from build123d import *

# Parameters (mm, degrees)
SKETCH1_W           = 62
SKETCH1_H           = 46
BOSS_EXTRUDE1_DEPTH = 5
SKETCH2_W           = 2
SKETCH2_H           = 5
SKETCH2_H_2         = 9
SKETCH2_H_3         = 32
SKETCH2_W_2         = 5
SKETCH2_H_4         = 2
BOSS_EXTRUDE2_DEPTH = 8
SKETCH3_W           = 17
SKETCH3_H           = 32
BOSS_EXTRUDE3_DEPTH = 1.5
SKETCH4_W           = 7
SKETCH4_H           = 5
BOSS_EXTRUDE4_DEPTH = 2.5


with BuildPart() as part:
    # Sketch1 → Boss-Extrude1 (new body)
    with BuildSketch(Plane(origin=(0, 0, 0), x_dir=(1, 0, 0), z_dir=(0, 1, 0))):
        with Locations((4.368421053, -7.717105263)):
            Rectangle(SKETCH1_W, SKETCH1_H)
    extrude(amount=BOSS_EXTRUDE1_DEPTH)

    # Sketch2 → Boss-Extrude2 (add)
    with BuildSketch(Plane(origin=(0, 5, 0), x_dir=(1, 0, 0), z_dir=(0, 1, 0))):
        with Locations((-20.631578947, 3.782894737)):
            Rectangle(SKETCH2_W, SKETCH2_H)
        with Locations((-20.631578947, -19.217105263)):
            Rectangle(SKETCH2_W, SKETCH2_H)
        Polygon((7.368421053, -23.717105263), (8.368421053, -22.717105263), (2.368421053, -16.717105263), (1.368421053, -17.717105263), align=None)
        with Locations((30.368421053, 6.782894737)):
            Rectangle(SKETCH2_W, SKETCH2_H_2)
        with Locations((30.368421053, -7.717105263)):
            Rectangle(SKETCH2_W, SKETCH2_H_2)
        with Locations((30.368421053, -22.217105263)):
            Rectangle(SKETCH2_W, SKETCH2_H_2)
        with Locations((10.368421053, -7.717105263)):
            Rectangle(SKETCH2_W, SKETCH2_H_3)
        with Locations((25.368421053, -7.717105263)):
            Rectangle(SKETCH2_W, SKETCH2_H_3)
        with Locations((-6.131578947, -24.717105263)):
            Rectangle(SKETCH2_W_2, SKETCH2_H_4)
    extrude(amount=BOSS_EXTRUDE2_DEPTH)

    # Sketch3 → Boss-Extrude3 (add)
    with BuildSketch(Plane(origin=(0, 13, 0), x_dir=(1, 0, 0), z_dir=(0, 1, 0))):
        with Locations((17.868421053, -7.717105263)):
            Rectangle(SKETCH3_W, SKETCH3_H)
    extrude(amount=BOSS_EXTRUDE3_DEPTH)

    # Sketch4 → Boss-Extrude4 (add)
    with BuildSketch(Plane(origin=(0, 14.5, 0), x_dir=(1, 0, 0), z_dir=(0, 1, 0))):
        with Locations((17.868421053, -21.217105263)):
            Rectangle(SKETCH4_W, SKETCH4_H)
    extrude(amount=BOSS_EXTRUDE4_DEPTH)


solid = part.part
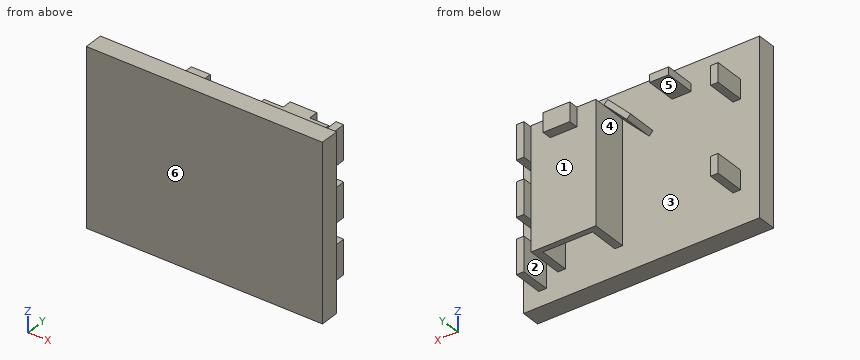
Check sheet for the modelled part. Datum: model origin and axes. Units: mm. Face numbers are marked on the shaded views. A direction names the side the tool comes from. Give positions to 0.01 mm unless a question says otherwise; leave off trailing zeros. Write each loop counter-clockwise with the first axis right and the second up, starting at its lowest first coordinate (ties: lowest second). Pieces come first, ordered by that corner, then holes. Notation, with made-up numbers: (1.5, 3.25) -> (30.5, 3.25) arc R14 cw to (30.5, 19.25) -> close; hole circle Ø10 at (21.25, 76.5). An arc over 180 degrees is marked (long way). Use one line per item in the form item = value. Start each with the question number.
1. Go/stop test with flat-tipped pins: P1, Ø2, axis at x = 6.5, z = 20, coming from the +Y side; P2, Ø2, axis at y = 16, z = 22, coming from the -X side; P3, Ø4, axis at y = 9, z = 18.5, coming from the +X side. Record where each tip stops, or that it passes through.
2. Section check B-B (z = -5.5). Record the cut outline in (x, y).
3. Access from +Z, -Z, +X, -X, +Y, -Y to the whole of each face (thin tool, end or side, straight path). Record for the marked faces 4, 5 and 6.
4. Section check D-D (z = 7). Record the cut outline in (x, y).
5. Section check C-C (y = 5.75). Count the separate pieces of the cut face and the enclosed holes in it, and give its area (3 significant figures).
6. Thickness scan on line 1 along Z through (x, y) = (29.5, 6.5); line 2 along X through (y, z) = (10, -4.5); line 3 along Y through (x, z) = (16, 4). Record the ranges inside material, lowest first. Write a range as from..to.
7. Mould release check, pull along X, two halves, no side actions. Record for the marked faces 1, 2 and 3: pulls with the +X half, pulls with the -X half, needs draft (parallel to the pull), parting line crosses it, or undercut.
8. Section check A-A (x = 20). Record the cut outline in (y, z).
Conclusion:
q1.P1 = 13
q1.P2 = 14.37
q1.P3 = 31.37
q2.outline = (-26.63, 0) -> (35.37, 0) -> (35.37, 5) -> (31.37, 5) -> (31.37, 13) -> (29.37, 13) -> (29.37, 5) -> (26.37, 5) -> (26.37, 14.5) -> (9.37, 14.5) -> (9.37, 5) -> (-19.63, 5) -> (-19.63, 13) -> (-21.63, 13) -> (-21.63, 5) -> (-26.63, 5) -> close; hole (11.37, 5) -> (24.37, 5) -> (24.37, 13) -> (11.37, 13) -> close
q3.face_4 = +Z, -Z, +Y
q3.face_5 = -Z, -X, +Y
q3.face_6 = +Z, -Z, +X, -X, -Y
q4.outline = (-26.63, 0) -> (35.37, 0) -> (35.37, 5) -> (31.37, 5) -> (31.37, 13) -> (29.37, 13) -> (29.37, 5) -> (26.37, 5) -> (26.37, 14.5) -> (9.37, 14.5) -> (9.37, 5) -> (-26.63, 5) -> close; hole (11.37, 5) -> (24.37, 5) -> (24.37, 13) -> (11.37, 13) -> close
q5.separate_pieces = 9
q5.enclosed_holes = 0
q5.area = 224 mm²
q6.line_1 = -11.28..-2.28, 3.22..12.22, 17.72..26.72
q6.line_2 = -21.63..-19.63, 9.37..11.37, 24.37..26.37, 29.37..31.37
q6.line_3 = 0..5, 13..14.5
q7.face_1 = needs draft
q7.face_2 = undercut
q7.face_3 = undercut
q8.outline = (0, -15.28) -> (5, -15.28) -> (5, 30.72) -> (0, 30.72) -> close; (13, -8.28) -> (14.5, -8.28) -> (14.5, 18.72) -> (17, 18.72) -> (17, 23.72) -> (13, 23.72) -> close
